The listing builds one solid part. Answer for the finished solid, in the listing's coordinates (mm). Face numbers are marked on the shaded views. A direction names the side the tool comes from. Round coordinates to 2 decimals unless told otherwise and drop trailing zeros. Write each loop counter-clockwise with the first axis right and the second up, starting at its lowest first coordinate (ties: lowest second). Pieces come first, ordered by that corner, then holes.
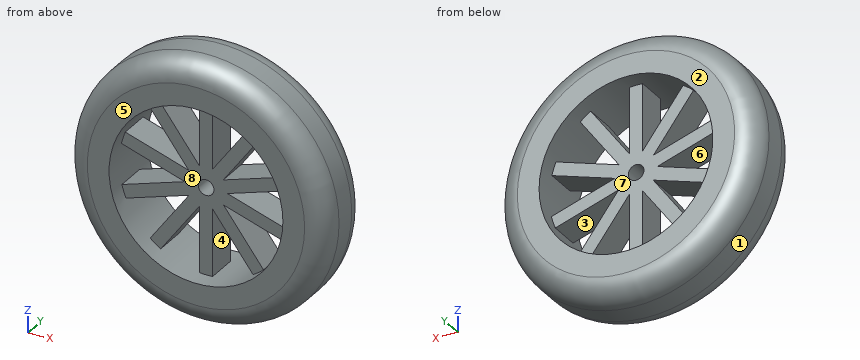
from build123d import *

# Parameters (mm, degrees)
F2_DEPTH = 3.5
F0_R     = 30
F0_R_2   = 20
F3_DEPTH = 7.5
F4_R     = 4.000000066
F4_R_2   = 1.8
F5_DEPTH = 3.5
F6_R     = 5
F7_R     = 5


with BuildPart() as f2:
    # F1 (on Front) → F2 (new body, symmetric)
    with BuildSketch(Plane.XZ):
        Polygon((-1.5, -23.2615247369), (1.5, -23.2615247369), (1.5, -4.4813106249), (0.0279501338, -2.5287712352), (-1.5, -4.6514858813), align=None)
        Polygon((0.0279501338, -2.5287712352), (1.5, -4.4813106249), (1.5, -2.0360415442), (0.5866393147, -1.7526086625), align=None)
        Polygon((1.5, -2.0360415442), (1.5, -4.4813106249), (12.8056726102, -19.4772503728), (15.2011628307, -17.6712529742), (3.9979355773, -2.8111976138), align=None)
        Polygon((-12.3720384359, -19.755535883), (-1.5, -4.6514858813), (-1.5, -2.0838847412), (-3.9348229661, -2.8988772188), (-14.806861402, -18.0029272205), align=None)
        Polygon((-1.5, -2.0838847412), (-1.5, -4.6514858813), (0.0279501338, -2.5287712352), (-0.5477580826, -1.7651469889), align=None)
        Polygon((1.5, -1.0797142258), (1.5, -2.0360415442), (3.9979355773, -2.8111976138), (2.4522419174, -0.7609764734), align=None)
        Polygon((-3.9348229661, -2.8988772188), (-1.5, -2.0838847412), (-1.5, -1.1050855059), (-2.4348229661, -0.8149924776), align=None)
        Polygon((2.4522419174, -0.7609764734), (3.9979355773, -2.8111976138), (21.7718478308, -8.3267745926), (22.660977137, -5.4615609746), (4.8870648835, 0.0540160042), align=None)
        Polygon((-21.5824822139, -8.8059635798), (-3.9348229661, -2.8988772188), (-2.4348229661, -0.8149924776), (-4.8870648835, -0.0540160042), (-22.5347241314, -5.9611023652), align=None)
        Polygon((1.8630056265, 0.0205915252), (2.4522419174, -0.7609764734), (4.8870648835, 0.0540160042), (2.4348229661, 0.8149924776), align=None)
        Polygon((-4.8870648835, -0.0540160042), (-2.4348229661, -0.8149924776), (-1.8630056265, -0.0205915252), (-2.4522419174, 0.7609764734), align=None)
        Polygon((2.4348229661, 0.8149924776), (4.8870648835, 0.0540160042), (22.5347241314, 5.9611023652), (21.5824822139, 8.8059635798), (3.9348229661, 2.8988772188), align=None)
        Polygon((-22.660977137, 5.4615609746), (-4.8870648835, -0.0540160042), (-2.4522419174, 0.7609764734), (-3.9979355773, 2.8111976138), (-21.7718478308, 8.3267745926), align=None)
        Polygon((1.5, 2.0838847412), (1.5, 1.1050855059), (2.4348229661, 0.8149924776), (3.9348229661, 2.8988772188), align=None)
        Polygon((-2.4522419174, 0.7609764734), (-1.5, 1.0797142258), (-1.5, 2.0360415442), (-3.9979355773, 2.8111976138), align=None)
        Polygon((0.5477580826, 1.7651469889), (1.5, 2.0838847412), (1.5, 4.6514858813), (-0.0279501338, 2.5287712352), align=None)
        Polygon((1.5, 4.6514858813), (1.5, 2.0838847412), (3.9348229661, 2.8988772188), (14.806861402, 18.0029272205), (12.3720384359, 19.755535883), align=None)
        Polygon((-3.9979355773, 2.8111976138), (-1.5, 2.0360415442), (-1.5, 4.4813106249), (-12.8056726102, 19.4772503728), (-15.2011628307, 17.6712529742), align=None)
        Polygon((-1.5, 4.4813106249), (-1.5, 2.0360415442), (-0.5866393147, 1.7526086625), (-0.0279501338, 2.5287712352), align=None)
        Polygon((-0.0279501338, 2.5287712352), (1.5, 4.6514858813), (1.5, 23.2615247369), (-1.5, 23.2615247369), (-1.5, 4.4813106249), align=None)
    extrude(amount=F2_DEPTH, both=True)

    # F0 (on Front) → F3 (join, symmetric)
    with BuildSketch(Plane.XZ):
        Circle(F0_R)
        Circle(F0_R_2, mode=Mode.SUBTRACT)
    extrude(amount=F3_DEPTH, both=True)

    # F4 (on Front) → F5 (join, symmetric)
    with BuildSketch(Plane.XZ):
        Circle(F4_R)
        Circle(F4_R_2, mode=Mode.SUBTRACT)
    extrude(amount=F5_DEPTH, both=True)

    # F6
    f6_edges = [f2.edges().sort_by_distance(p)[0] for p in [
        (-30, -7.5, 0),
    ]]
    fillet(f6_edges, radius=F6_R)

    # F7
    f7_edges = [f2.edges().sort_by_distance(p)[0] for p in [
        (-30, 7.5, 0),
    ]]
    fillet(f7_edges, radius=F7_R)


solid = f2.part
1. For a pull along X with two mould halves and no side action, classify the marked faces 1, 2, 3 and 4 as released by +X, released by -X, zero draft, split by the parting line, or undercut.
Geometry says:
face 1: split by the parting line
face 2: zero draft
face 3: undercut
face 4: undercut
2. Section B-B on y = 1.75 is taken. Give the number of separate pieces and of enclosed holes in the cut face, plus the area to 3 significant figures.
Geometry says:
separate pieces: 1
enclosed holes: 11
area: 2,090 mm2
3. Straight lines are drawn through the part: line 1 along Z through (x, y) = (-15.5, -3.25); line 2 along Z through (x, y) = (-15, 1.25); line 3 along Z through (x, y) = (0, 0.75). For each, find the intervals that lie inside material, in ascending order.
Geometry says:
line 1: z = -25.62 to -12.64, -6.77 to -3.61, 3.24 to 6.38, 12.64 to 25.62
line 2: z = -25.98 to -13.23, -6.6 to -3.44, 3.08 to 6.23, 13.23 to 25.98
line 3: z = -30 to -1.8, 1.8 to 30
4. Given pin 1 (2 mm diameter, centred on x = -6.5, y = -1, fed in from -Z); pin 2 (7.5 mm diameter, centred on y = -1, z = 13.5, fed in from +X); pin 3 (8 mm diameter, centred on y = 4, z = -7, fed in from +X), each flat-ended and moving along its own axis, determine where each tip first touches the part or whether it passes through.
Geometry says:
pin 1: stops at z = -29.49
pin 2: stops at x = 28.37
pin 3: stops at x = 29.82
5. Section A-A on x = 0 is taken. Determine the outline of the cut face in (y, z), plus the area to 3 significant figures.
Geometry says:
outline: (-7.5, -25) arc R5 ccw to (-2.5, -30) - (2.5, -30) arc R5 ccw to (7.5, -25) - (7.5, -20) - (3.5, -20) - (3.5, -1.8) - (-3.5, -1.8) - (-3.5, -20) - (-7.5, -20) - close; (-7.5, 20) - (-3.5, 20) - (-3.5, 1.8) - (3.5, 1.8) - (3.5, 20) - (7.5, 20) - (7.5, 25) arc R5 ccw to (2.5, 30) - (-2.5, 30) arc R5 ccw to (-7.5, 25) - close
area: 533 mm2
6. A tool of negligible diameter and unlimited length cuts with its end or side. For the marked faces 5, 6, 7 and 8, from which of +Z, -Z, +X, -X, +Y, -Y can it reach the whole face along a straight path? Write none if from no direction.
Geometry says:
face 5: +Z, -Z, +X, -X, -Y
face 6: +Y, -Y
face 7: +Y
face 8: -Y
